Here's how the part is built. I have some questions about the finished solid (model axes, mm). A direction names the side the tool comes from. Coordinates: 2 decimals unless noted, no trailing zeros. Order: outer loops, then holes, each group sorted by start corner. A loop starts at its lowest first (then second) coordinate and runs counter-clockwise, first axis right, second up. Notation, with made-up numbers: (-21, 62) - (3, 62) arc R18 cw to (3, 87) - close; hole circle Ø1 at (-1, 6.25). An arc over 180 degrees is marked (long way). Answer in a Markdown table with one row per item. Add a question column.
Item 1: I want a section at B-B (y = 14.5). Please give me the cut outline in (x, z), plus the area to 3 significant figures.
Item 2: Will these pins go through, and if not, where does the flat tip stop? pin 1 Ø3 at (y, z) = (14.5, 4) entering from +X; pin 2 Ø4.5 at (y, z) = (57.5, 7) entering from +X; pin 3 Ø7.5 at (y, z) = (57, -2) entering from -X.
Item 3: I want a section at A-A (x = -1). Please give me the cut outline in (y, z).
Item 4: Thinking about a two-plate mould opening in Y: for faces 1 (the cylindrical face through (46.54, 64.75, -6.57)), 2 (the flat face through (1, -49.25, -10)), 3 (the flat face through (-49, 60, 0)), which applies, +Y half, -Y half, draft (parallel to the pull), parting line (faces both ways), or undercut?
Item 5: On a 3-axis mill with a long thin cutter (end or side, diameter ignored), from which of +Z, -Z, +X, -X, +Y, -Y can I reach the whole of each face in a straight line? I mean faces 4 (the flat face through (-66, -1, 4)), 5 (the cylindrical face through (67.5, 47.82, -9.86)), 6 (the flat face through (47, 56, -8)). Say none if no direction works.
Item 6: If I drill on line 1 along X through (y, z) = (30, -1); line 2 along Z through (x, y) = (-46, 61); line 3 along Y through (x, z) = (-31.5, -15.5), over which ranges is the centre line in solid material (lowest first)? Write a range as from..to.
Item 7: I want a section at C-C (x = 37.5). Please give me the cut outline in (y, z), plus the area to 3 significant figures.
```python
from build123d import *

# Parameters (mm, degrees)
F1_DEPTH  = 20
F0_W      = 132
F0_H      = 92.5
F2_DEPTH  = 2
F0_W_2    = 128
F0_H_2    = 88.5
F3_DEPTH  = 6
F4_W      = 5
F4_H      = 10
F5_DEPTH  = 10
F7_DEPTH  = 5
F9_R      = 1.5
F10_DEPTH = 5


with BuildPart() as f1:
    # F0 (on Top) → F1 (new body)
    with BuildSketch(Plane.XY):
        with BuildLine():
            Line((71, -44.25), (71, 44.25))
            ThreePointArc((71, 44.25), (68.949747, 49.199747), (64, 51.25))
            Line((64, 51.25), (-64, 51.25))
            ThreePointArc((-64, 51.25), (-68.949747, 49.199747), (-71, 44.25))
            Line((-71, 44.25), (-71, -44.25))
            ThreePointArc((-71, -44.25), (-68.949747, -49.199747), (-64, -51.25))
            Line((-64, -51.25), (-20, -51.25))
            Line((-20, -51.25), (20, -51.25))
            Line((20, -51.25), (64, -51.25))
            ThreePointArc((64, -51.25), (68.949747, -49.199747), (71, -44.25))
        make_face()
        with BuildLine():
            Line((-64, 49.25), (64, 49.25))
            ThreePointArc((64, 49.25), (67.535534, 47.785534), (69, 44.25))
            Line((69, 44.25), (69, -44.25))
            ThreePointArc((69, -44.25), (67.535534, -47.785534), (64, -49.25))
            Line((64, -49.25), (-64, -49.25))
            ThreePointArc((-64, -49.25), (-67.535534, -47.785534), (-69, -44.25))
            Line((-69, -44.25), (-69, 44.25))
            ThreePointArc((-69, 44.25), (-67.535534, 47.785534), (-64, 49.25))
        make_face(mode=Mode.SUBTRACT)
    extrude(amount=-F1_DEPTH)

    # F0 (on Top) → F2 (join)
    with BuildSketch(Plane.XY):
        with BuildLine():
            Line((20, -59.75), (20, -51.25))
            Line((20, -51.25), (-20, -51.25))
            Line((-20, -51.25), (-20, -59.75))
            ThreePointArc((-20, -59.75), (-18.535534, -63.285534), (-15, -64.75))
            Line((-15, -64.75), (15, -64.75))
            ThreePointArc((15, -64.75), (18.535534, -63.285534), (20, -59.75))
        make_face()
        with BuildLine():
            Line((71, -44.25), (71, 44.25))
            ThreePointArc((71, 44.25), (68.949747, 49.199747), (64, 51.25))
            Line((64, 51.25), (-64, 51.25))
            ThreePointArc((-64, 51.25), (-68.949747, 49.199747), (-71, 44.25))
            Line((-71, 44.25), (-71, -44.25))
            ThreePointArc((-71, -44.25), (-68.949747, -49.199747), (-64, -51.25))
            Line((-64, -51.25), (-20, -51.25))
            Line((-20, -51.25), (20, -51.25))
            Line((20, -51.25), (64, -51.25))
            ThreePointArc((64, -51.25), (68.949747, -49.199747), (71, -44.25))
        make_face()
        with BuildLine():
            Line((-64, 49.25), (64, 49.25))
            ThreePointArc((64, 49.25), (67.535534, 47.785534), (69, 44.25))
            Line((69, 44.25), (69, -44.25))
            ThreePointArc((69, -44.25), (67.535534, -47.785534), (64, -49.25))
            Line((64, -49.25), (-64, -49.25))
            ThreePointArc((-64, -49.25), (-67.535534, -47.785534), (-69, -44.25))
            Line((-69, -44.25), (-69, 44.25))
            ThreePointArc((-69, 44.25), (-67.535534, 47.785534), (-64, 49.25))
        make_face(mode=Mode.SUBTRACT)
        with BuildLine():
            ThreePointArc((69, 44.25), (67.535534, 47.785534), (64, 49.25))
            Line((64, 49.25), (-64, 49.25))
            ThreePointArc((-64, 49.25), (-67.535534, 47.785534), (-69, 44.25))
            Line((-69, 44.25), (-69, -44.25))
            ThreePointArc((-69, -44.25), (-67.535534, -47.785534), (-64, -49.25))
            Line((-64, -49.25), (64, -49.25))
            ThreePointArc((64, -49.25), (67.535534, -47.785534), (69, -44.25))
            Line((69, -44.25), (69, 44.25))
        make_face()
        Rectangle(F0_W, F0_H, mode=Mode.SUBTRACT)
    extrude(amount=F2_DEPTH)

    # F0 (on Top) → F3 (join)
    with BuildSketch(Plane.XY):
        Rectangle(F0_W, F0_H)
        Rectangle(F0_W_2, F0_H_2, mode=Mode.SUBTRACT)
    extrude(amount=F3_DEPTH)

    # F4 (on face) → F5 (join)
    with BuildSketch(Plane(origin=(0, 51.25, 0), x_dir=(-1, 0, 0), z_dir=(0, 1, 0))):
        with Locations((-46.5, -3)):
            Rectangle(F4_W, F4_H)
    extrude(amount=F5_DEPTH)

    # F6 (on face) → F7 (join)
    with BuildSketch(Plane.YZ.offset(49)):
        with BuildLine():
            Line((61.25, 2), (61.25, -8))
            ThreePointArc((61.25, -8), (64.785534, -6.535534), (66.25, -3))
            Line((66.25, -3), (66.25, 7))
            ThreePointArc((66.25, 7), (64.785534, 10.535534), (61.25, 12))
            Line((61.25, 12), (61.25, 8.5))
            ThreePointArc((61.25, 8.5), (62.31066, 8.06066), (62.75, 7))
            ThreePointArc((62.75, 7), (62.31066, 5.93934), (61.25, 5.5))
            Line((61.25, 5.5), (61.25, 2))
        make_face()
        with BuildLine():
            Line((56.25, 2), (61.25, 2))
            Line((61.25, 2), (61.25, 5.5))
            ThreePointArc((61.25, 5.5), (59.75, 7), (61.25, 8.5))
            Line((61.25, 8.5), (61.25, 12))
            ThreePointArc((61.25, 12), (57.714466, 10.535534), (56.25, 7))
            Line((56.25, 7), (56.25, 2))
        make_face()
    extrude(amount=-F7_DEPTH)

    # F9 (on offset) → F10 (join)
    with BuildSketch(Plane.YZ.offset(-49)):
        with BuildLine():
            Line((56.25, 2), (51.25, 2))
            Line((51.25, 2), (51.25, -8))
            Line((51.25, -8), (61.25, -8))
            ThreePointArc((61.25, -8), (64.785534, -6.535534), (66.25, -3))
            Line((66.25, -3), (66.25, 7))
            ThreePointArc((66.25, 7), (61.25, 12), (56.25, 7))
            Line((56.25, 7), (56.25, 2))
        make_face()
        with Locations((61.25, 7)):
            Circle(F9_R, mode=Mode.SUBTRACT)
    extrude(amount=F10_DEPTH)


solid = f1.part
```
Values follow:
| question | item | result |
|---|---|---|
| 1 | outline | (-71, -20) - (-69, -20) - (-69, 0) - (-64, 0) - (-64, 6) - (-66, 6) - (-66, 2) - (-71, 2) - close; (64, 0) - (69, 0) - (69, -20) - (71, -20) - (71, 2) - (66, 2) - (66, 6) - (64, 6) - close |
| 1 | area | 124 mm^2 |
| 2 | pin 1 | stops at x = 66 |
| 2 | pin 2 | stops at x = 49 |
| 2 | pin 3 | stops at x = -49 |
| 3 | outline | (-64.75, 0) - (-51.25, 0) - (-51.25, -20) - (-49.25, -20) - (-49.25, 0) - (-44.25, 0) - (-44.25, 6) - (-46.25, 6) - (-46.25, 2) - (-64.75, 2) - close; (44.25, 0) - (49.25, 0) - (49.25, -20) - (51.25, -20) - (51.25, 2) - (46.25, 2) - (46.25, 6) - (44.25, 6) - close |
| 4 | face 1 | +Y half |
| 4 | face 2 | undercut |
| 4 | face 3 | draft |
| 5 | face 4 | +Z, -X, +Y, -Y |
| 5 | face 5 | -Z |
| 5 | face 6 | -Z, +X, -X, +Y |
| 6 | line 1 | x = -71..-69, 69..71 |
| 6 | line 2 | z = -8..5.52, 8.48..11.99 |
| 6 | line 3 | y = -51.25..-49.25, 49.25..51.25 |
| 7 | outline | (-51.25, -20) - (-49.25, -20) - (-49.25, 0) - (-44.25, 0) - (-44.25, 6) - (-46.25, 6) - (-46.25, 2) - (-51.25, 2) - close; (44.25, 0) - (49.25, 0) - (49.25, -20) - (51.25, -20) - (51.25, 2) - (46.25, 2) - (46.25, 6) - (44.25, 6) - close |
| 7 | area | 124 mm^2 |
